CAD build for the part. Positions are in the model's coordinates, mm. Face numbers are marked on the shaded views. A direction names the side the tool comes from. Give positions to 0.01 mm unless a question says otherwise; leave off trailing zeros. Write each loop counter-clockwise with the first axis right and the second up, starting at its lowest first coordinate (ties: lowest second). Pieces come first, ordered by that corner, then holes. Notation, with made-up numbers: (72, -1) - (82, -1) arc R17 cw to (82, 23) - close; hole circle Ø2 at (-3.75, -35.5). An arc over 180 degrees is marked (long way). Put each result on its own line as item: value. Start each with the question number.
1. Tool access for the marked faces 1 and 2: list every direction of +Z, -Z, +X, -X, +Y, -Y with a clear straight run to the whole face (end or side of a thin tool).
2. Cut at C-C on x = 28.75. List the corners of the cut face in (y, z).
3. Cut at D-D on y = 36.5. List the corners of the cut face in (x, z).
4. Cut at A-A on x = 37.5. List the corners of the cut face in (y, z).
5. Wall check: line 1 (Z direction, x = 36.25, y = 34.8); line 2 (Y direction, x = 37.5, z = -5.3); line 3 (Y direction, x = 31.25, z = -3.75). Give the ranges that are in metal, low to high.
6. Cut at B-B on y = 33.4. List the corners of the cut face in (x, z), and give its area (3 significant figures).
7. Drop flat-ended pins along their axis: pin 1 (2 mm diameter, centred on y = 37.5, z = -5, fed in from +X); pin 2 (2 mm diameter, centred on x = 31, z = -2, fed in from -Y); pin 3 (1 mm diameter, centred on x = 29, z = -2.5, fed in from -Y). Give the stop position or say it passes through.
8. Mould opens along X. For the marked faces 3, 4 and 5 say: +X half, -X half, draft (parallel to the pull), parting line (faces both ways), or undercut.
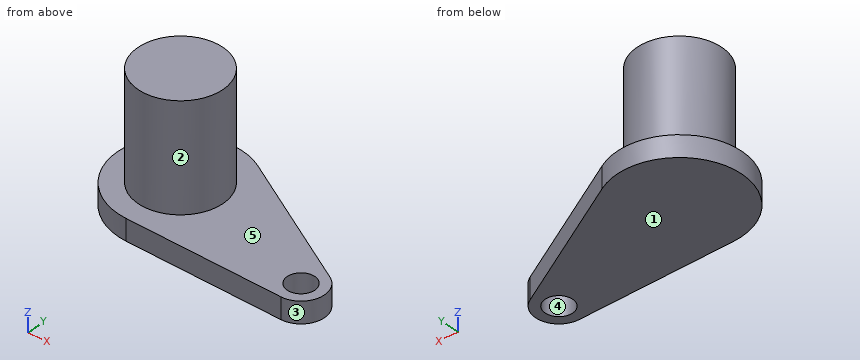
from build123d import *

# Parameters (mm, degrees)
SKETCH1_R               = 2
BOSS_EXTRUDE1_DEPTH     = 5
BOSS_EXTRUDE2_DEPTH     = 1
CUT_EXTRUDE1_DEPTH      = 56.072597377
CUT_EXTRUDE1_DEPTH_BACK = 56.072597377
SKETCH3_R               = 0.65


# Read off the part's stored shape, not the designer's step: Boss-Extrude2
with BuildPart() as part:
    # Sketch1 → Boss-Extrude1 (new body)
    with BuildSketch(Plane.XY):
        with Locations((30.458296942, 35.732918139)):
            Circle(SKETCH1_R)
    extrude(amount=-BOSS_EXTRUDE1_DEPTH)

    # Boss-Extrude2 outline → Boss-Extrude2 (add)
    with BuildSketch(Plane(origin=(0, 0, -5), x_dir=(-1, 0, 0), z_dir=(0, 0, -1))):
        with BuildLine():
            ThreePointArc((-38.30710157, 34.824835399), (-38.848941129, 33.586198742), (-37.781773498, 32.756160115))
            Line((-37.781773498, 32.756160115), (-30.446238276, 32.786178641))
            ThreePointArc((-30.446238276, 32.786178641), (-27.603676035, 36.464053256), (-31.864257159, 38.32264688))
            Line((-31.864257159, 38.32264688), (-38.30710157, 34.824835399))
        make_face()
    extrude(amount=BOSS_EXTRUDE2_DEPTH)

    # Sketch3 → Cut-Extrude1 (cut, two sides: drawn at the far end of the back side and taken through both)
    with BuildSketch(Plane.XY.offset(-5).offset(-CUT_EXTRUDE1_DEPTH_BACK)):
        with Locations((37.781773498, 33.857199764)):
            Circle(SKETCH3_R)
    extrude(amount=CUT_EXTRUDE1_DEPTH + CUT_EXTRUDE1_DEPTH_BACK, mode=Mode.SUBTRACT)


solid = part.part
Report:
1. face 1: -Z, +X, -X, +Y, -Y
1. face 2: +Z
2. outline: (33.33, -6) - (38.13, -6) - (38.13, -5) - (36.77, -5) - (36.77, 0) - (34.69, 0) - (34.69, -5) - (33.33, -5) - close
3. outline: (27.61, -6) - (35.22, -6) - (35.22, -5) - (32.31, -5) - (32.31, 0) - (28.61, 0) - (28.61, -5) - (27.61, -5) - close
4. outline: (32.76, -6) - (33.27, -6) - (33.27, -5) - (32.76, -5) - close; (34.44, -6) - (35.26, -6) - (35.26, -5) - (34.44, -5) - close
5. line 1: z = -6 to -5
5. line 2: y = 32.76 to 33.27, 34.44 to 35.26
5. line 3: y = 33.9 to 37.57
6. outline: (28.66, -6) - (37.32, -6) - (37.32, -5) - (28.66, -5) - close; (38.24, -6) - (38.78, -6) - (38.78, -5) - (38.24, -5) - close
6. area: 9.20 mm²
7. pin 1: stops at x = 35.22
7. pin 2: stops at y = 33.73
7. pin 3: stops at y = 33.98
8. face 3: +X half
8. face 4: undercut
8. face 5: draft
